Build history of the part. All positions in model axes, mm. Face numbers are marked on the shaded views. A direction names the side the tool comes from. Round coordinates to 2 decimals unless told otherwise and drop trailing zeros. Write each loop counter-clockwise with the first axis right and the second up, starting at its lowest first coordinate (ties: lowest second). Pieces come first, ordered by that corner, then holes.
1) Saw through at A-A (y = -0.1). Write the cut outline in (x, z).
2) Pull direction Z, two halves, no side cores. Call the marked faces 1, 2 and 3: +Z half, -Z half, draft (parallel to the pull), parting line (faces both ways), or undercut.
3) Which spindle directions (+Z, -Z, +X, -X, +Y, -Y) get a long thin tool onto all of the face, cutting with end or side? Do the marked faces 4, 5 and 6. Say none if no direction does.
4) Saw through at C-C (z = 9). State how many separate pieces and enclosed holes the cut face has, plus the area to 3 significant figures.
5) Saw through at B-B (x = 10.25). Write the cut outline in (y, z), plus the area to 3 significant figures.
6) Wall check: probe 1 along X at (y, z) = (0.35, -5); probe 2 along Z at (x, y) = (8.5, -1.3); probe 3 along X at (y, z) = (0.9, -6.25). Give the ranges that are in metal, low to high.
Autodesk Inventor part; units mm, degrees
ref_plane "YZ Plane" through (0, 0, 0) normal (1, 0, 0) x (0, 1, 0)
ref_plane "XZ Plane" through (0, 0, 0) normal (0, 1, 0) x (-1, 0, 0)
ref_plane "XY Plane" through (0, 0, 0) normal (0, 0, 1) x (1, 0, 0)
sketch "Sketch1" plane through (0, 0, 0) normal (0, 1, 0) x (-1, 0, 0)
  line L0 (14, 12) -> (-14, 12)
  line L1 (-14, 12) -> (-14, -8)
  line L2 (-14, -8) -> (14, -8)
  line L3 (14, -8) -> (14, 12)
  point P0 (0, 0)
  dimension "d0" = 28
  dimension "d1" = 20
  dimension "d4" = 14
extrude "Extrusion1" add sketch "Sketch1" along normal mid plane 4
sketch "Sketch2" plane through (-14, 2, 12) normal (0, 0, 1) x (1, 0, 0)
  line L0 (0, 0) -> (28, 0)
  line L1 (14, 0) -> (12.9393, -1.0607)
  line L2 (14, 0) -> (15.5, 0) construction
  line L3 (12.9393, -1.0607) -> (11.8787, 0)
  line L4 (11.8787, 0) -> (10.818, -1.0607)
  line L5 (10.818, -1.0607) -> (9.7574, 0)
  line L6 (9.7574, 0) -> (8.6967, -1.0607)
  line L7 (8.6967, -1.0607) -> (7.636, 0)
  line L8 (7.636, 0) -> (6.5754, -1.0607)
  line L9 (6.5754, -1.0607) -> (5.5147, 0)
  line L10 (5.5147, 0) -> (4.4541, -1.0607)
  line L11 (4.4541, -1.0607) -> (3.3934, 0)
  line L12 (3.3934, 0) -> (2.3327, -1.0607)
  line L13 (2.3327, -1.0607) -> (1.2721, 0)
  line L14 (1.2721, 0) -> (0, -1.2721)
  line L15 (0, -4) -> (0, 0)
  line L16 (14, 0) -> (15.0607, -1.0607)
  line L17 (15.0607, -1.0607) -> (16.1213, 0)
  line L18 (16.1213, 0) -> (17.182, -1.0607)
  line L19 (17.182, -1.0607) -> (18.2426, 0)
  line L20 (18.2426, 0) -> (19.3033, -1.0607)
  line L21 (19.3033, -1.0607) -> (20.364, 0)
  line L22 (20.364, 0) -> (21.4246, -1.0607)
  line L23 (21.4246, -1.0607) -> (22.4853, 0)
  line L24 (22.4853, 0) -> (23.5459, -1.0607)
  line L25 (23.5459, -1.0607) -> (24.6066, 0)
  line L26 (24.6066, 0) -> (25.6673, -1.0607)
  line L27 (25.6673, -1.0607) -> (26.7279, 0)
  line L28 (26.7279, 0) -> (28, -1.2721)
  line L29 (28, -4) -> (28, 0)
  point P0 (14, -2)
  point P1 (1.2721, 0)
  point P2 (1.2721, 0)
  point P3 (5.5147, 0)
  point P4 (5.5147, 0)
  point P5 (7.636, 0)
  point P6 (7.636, 0)
  point P7 (9.7574, 0)
  point P8 (9.7574, 0)
  dimension "d5" = 1.5
  dimension "d6" = 135
  dimension "d7" = 1.5
extrude "Extrusion2" cut sketch "Sketch2" against normal blind 50
mirror "Mirror1" about plane through (0, 0, 0) normal (0, 1, 0) of "Extrusion2"
sketch "Sketch4" plane through (0, 0, 0) normal (0, 1, 0) x (-1, 0, 0)
  circle A0 centre (9.757, -5) radius 2
  circle A1 centre (-9.757, -5) radius 2
  circle A2 centre (-9.757, 9) radius 2
  circle A3 centre (9.757, 9) radius 2
  point P0 (0, 0)
  dimension "d14" = 4
  dimension "d15" = 4
  dimension "d16" = 4
  dimension "d17" = 4
extrude "Extrusion4" cut sketch "Sketch4" against normal mid plane 6
properties part number "g2Tensioner"
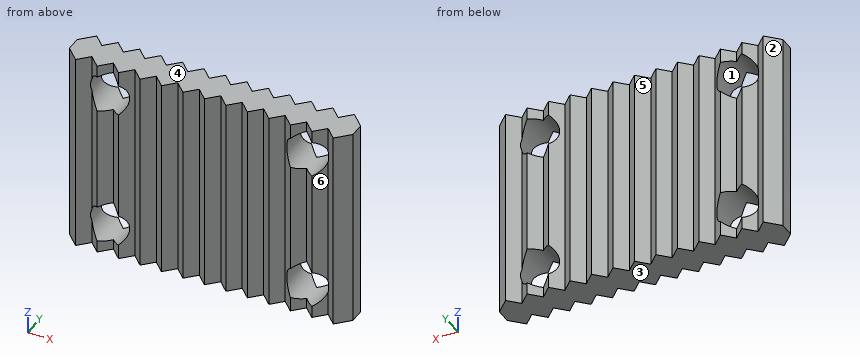
Evaluation:
1. outline: (-14, -8) - (14, -8) - (14, 12) - (-14, 12) - close; hole circle Ø4 at (-9.76, -5); hole circle Ø4 at (-9.76, 9); hole circle Ø4 at (9.76, -5); hole circle Ø4 at (9.76, 9)
2. face 1: undercut
2. face 2: draft
2. face 3: -Z half
3. face 4: +Z, +X, -X, +Y, -Y
3. face 5: +Z, -Z, +Y
3. face 6: +Z, -Z, -Y
4. separate pieces: 3
4. enclosed holes: 0
4. area: 57.9 mm2
5. outline: (-1.64, -8) - (1.64, -8) - (1.64, -6.94) - (-1.64, -6.94) - close; (-1.64, -3.06) - (1.64, -3.06) - (1.64, 7.06) - (-1.64, 7.06) - close; (-1.64, 10.94) - (1.64, 10.94) - (1.64, 12) - (-1.64, 12) - close
5. area: 40.3 mm2
6. probe 1: x = -14 to -11.76, -7.76 to 7.76, 11.76 to 14
6. probe 2: z = -8 to -6.56, -3.44 to 7.44, 10.56 to 12
6. probe 3: x = -13.83 to -11.32, -8.2 to 8.2, 11.32 to 13.83
